```python
from build123d import *

# Parameters (mm, degrees)
F3_R     = 3.95605
F4_DEPTH = 12.7
F6_R     = 1.3208
F7_DEPTH = 19.051


with BuildPart() as f1:
    # F0 (on Front) → F1 (revolve)
    with BuildSketch(Plane.XZ):
        with BuildLine():
            Line((0, 9.525), (0, -9.525))
            ThreePointArc((0, -9.525), (9.525, 0), (0, 9.525))
        make_face()
    revolve(axis=Axis((0, 0, 0), (0, 0, -1)))

    # F3 (on offset) → F4 (cut)
    with BuildSketch(Plane.XZ.offset(9.525)):
        Circle(F3_R)
    extrude(amount=-F4_DEPTH, mode=Mode.SUBTRACT)

    # F6 (on offset) → F7 (cut, through all)
    with BuildSketch(Plane.XY.offset(9.525)):
        Circle(F6_R)
    extrude(amount=-F7_DEPTH, mode=Mode.SUBTRACT)


solid = f1.part
```
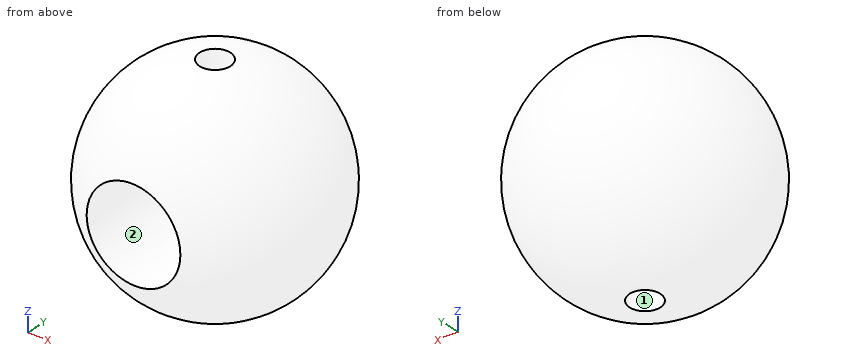
Model file for the job. Use its own axes, mm. Face numbers are marked on the shaded views. A direction names the side the tool comes from. Give positions to 0.01 mm unless a question says otherwise; leave off trailing zeros. Loops run counter-clockwise (first coordinate to the right, second up) from the corner with the lowest first, then second, coordinate; pieces in that order, holes last. Notation, with made-up numbers: (-14.5, -28.75) - (16.5, -28.75) arc R24 cw to (16.5, 1.25) - close; hole circle Ø5 at (26, 37). An arc over 180 degrees is marked (long way). One line per item, written item: value. Start each with the question number.
1. Which spindle directions (+Z, -Z, +X, -X, +Y, -Y) get a long thin tool onto all of the face, cutting with end or side? Do the marked faces 1 and 2. Say none if no direction does.
2. Slice it at D-D (z = 5). List the corners of the cut face in (x, y), plus the area to 3 significant figures.
3. Slice it at A-A (y = 0). List the corners of the cut face in (x, z) (3 decimals), plus the area to 3 significant figures.
4. Pin check, flat tips, straight feed: pin 1 (5 mm diameter, centred on x = 2.5, z = -7.5, fed in from -Y); pin 2 (6.5 mm diameter, centred on x = 0, z = 0, fed in from -Y) (3 decimals); pin 3 (10 mm diameter, centred on x = -1, z = -2.5, fed in from +Y) (3 decimals). Stop position of each tip, or through.
5. Slice it at C-C (z = 0). List the corners of the cut face in (x, y) (3 decimals), plus the area to 3 significant figures.
6. Probe L1, parallel to Y at x = 0.25, z = -7; L2, parallel to X at y = -0.5, z = -5.5; L3, parallel to X at y = 2, z = -3.5. List the from-to ranges inside material, lowest first. Write a range as from..to.
7. Slice it at B-B (x = 0). List the corners of the cut face in (y, z) (3 decimals).
Solution:
1. face 1: +Z, -Z
1. face 2: -Y
2. outline: circle Ø16.21 at (0, 0); hole circle Ø2.64 at (0, 0)
2. area: 201 mm^2
3. outline: (-1.321, -9.433) - (-1.321, -3.729) arc R3.956 cw to (-1.321, 3.729) - (-1.321, 9.433) arc R9.525 ccw to start; (1.321, -9.433) arc R9.525 ccw to (1.321, 9.433) - (1.321, 3.729) arc R3.956 cw to (1.321, -3.729) - close
3. area: 206 mm^2
4. pin 1: stops at y = -7.84
4. pin 2: stops at y = 3.175
4. pin 3: stops at y = 9.525
5. outline: (-3.956, -8.665) - (-3.956, 3.175) - (3.956, 3.175) - (3.956, -8.665) arc R9.525 ccw (long way) to start
5. area: 187 mm^2
6. L1: y = -6.45..-1.3, 1.3..6.45
6. L2: x = -7.76..-1.22, 1.22..7.76
6. L3: x = -8.63..-1.84, 1.84..8.63
7. outline: (-8.665, -3.956) arc R9.525 ccw to (-1.321, -9.433) - (-1.321, -3.956) - close; (-8.665, 3.956) - (-1.321, 3.956) - (-1.321, 9.433) arc R9.525 ccw to start; (1.321, -9.433) arc R9.525 ccw to (1.321, 9.433) - (1.321, 3.956) - (3.175, 3.956) - (3.175, -3.956) - (1.321, -3.956) - close
